The listing builds one solid part. Answer for the finished solid, in the listing's coordinates (mm). Give positions to 0.01 mm unless a question says otherwise; leave off trailing zeros. Order: outer loops, then holes, each group sorted by start corner. A loop starts at its lowest first (then second) coordinate and runs counter-clockwise, first axis right, second up. Notation, with made-up numbers: (54.5, 45) -> (88.5, 45) arc R23 cw to (88.5, 70) -> close; hole circle Ø6 at (82.5, 35.25). An arc over 180 degrees is marked (long way). Write item = value, one per line. Start each with the question number.
Autodesk Inventor part; units mm, degrees
ref_plane "YZ Plane" through (0, 0, 0) normal (1, 0, 0) x (0, 1, 0)
ref_plane "XZ Plane" through (0, 0, 0) normal (0, 1, 0) x (-1, 0, 0)
ref_plane "XY Plane" through (0, 0, 0) normal (0, 0, 1) x (1, 0, 0)
sketch "Sketch1" plane through (0, 0, 0) normal (0, 1, 0) x (-1, 0, 0)
  line L0 (-9.75, 149.5) -> (9.75, 149.5)
  line L1 (9.75, 149.5) -> (9.75, -149.5)
  line L2 (9.75, -149.5) -> (-9.75, -149.5)
  line L3 (-9.75, -149.5) -> (-9.75, 149.5)
  line L4 (-9.75, 149.5) -> (9.75, -149.5) construction
  line L5 (9.75, 149.5) -> (-9.75, -149.5) construction
  point P0 (0, 0)
  dimension "d0" = 19.5
  dimension "d1" = 299
extrude "Extrusion1" add sketch "Sketch1" along normal blind 5
chamfer "Chamfer1" distance 3 angle 45 1 edges at (-9.75, 5, 0)
sketch "Sketch2" plane through (-9.75, 0, 149.5) normal (0, 0, 1) x (1, 0, 0)
  line L0 (0, 2) -> (3, 5)
  line L1 (0, 0) -> (0, 2)
  line L2 (0, 0) -> (19.5, 0)
  line L3 (19.5, 0) -> (19.5, 5)
  line L4 (3, 5) -> (19.5, 5)
  line L5 (16.5, 4) -> (11.5, 4)
  line L6 (11.5, 4) -> (11.5, 1)
  line L7 (11.5, 1) -> (16.5, 1)
  line L8 (16.5, 1) -> (16.5, 4)
  line L9 (16.5, 4) -> (11.5, 1) construction
  line L10 (11.5, 4) -> (16.5, 1) construction
  point P0 (9.75, 0)
  point P1 (14, 2.5)
  point P2 (19.5, 2.5)
  dimension "d7" = 5
  dimension "d8" = 3
  dimension "d9" = 3
extrude "Extrusion2" cut sketch "Sketch2" against normal blind 7.1 contours L8 L7 L6 L5
sketch "Sketch3" plane through (9.75, 0, -149.5) normal (0, 0, -1) x (-1, 0, 0)
  line L0 (8, 1) -> (8, 4)
  line L1 (3, 1) -> (8, 1)
  line L2 (3, 4) -> (3, 1)
  line L3 (8, 4) -> (3, 4)
  line L4 (7.8, 1.2) -> (7.8, 3.8)
  line L5 (7.8, 3.8) -> (3.2, 3.8)
  line L6 (3.2, 3.8) -> (3.2, 1.2)
  line L7 (3.2, 1.2) -> (7.8, 1.2)
  point P0 (9.75, 0)
  dimension "d12" = 0.2
extrude "Extrusion3" add sketch "Sketch3" along normal blind 7 contours L7 L6 L5 L4
properties part number "SEPARADOR" material "Steel, Mild, Welded"
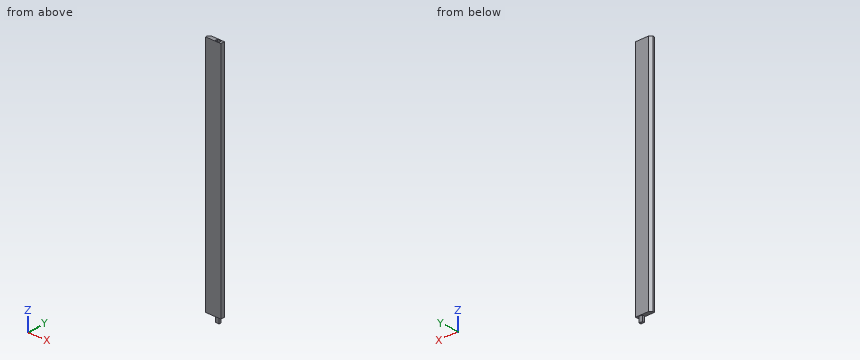
Item 1: A cutting plane is placed at B-B, the plane z = -105.5. Write down the section's boundary in (x, y).
Item 2: Consider L1, parallel to Z at x = -7.75, y = 3.3; L2, parallel to Z at x = 3, y = 1.3; L3, parallel to X at y = 3.1, z = 29.5. Determine where each line is inside the solid, lowest interval first. Write a range as from..to.
Item 3: Flat-ended cylindrical pins translate along their axes: pin 1 (2.5 mm diameter, centred on x = 5, z = -153.5, fed in from +Y); pin 2 (0.8 mm diameter, centred on y = 2, z = -152.5, fed in from -X); pin 3 (3 mm diameter, centred on y = 4, z = -19, fed in from -X). Find the tip coordinate at first contact, or state that the pin passes through.
Item 4: A cutting plane is placed at A-A, the plane y = 2.95. Write down the section's boundary in (x, z), plus the area to 3 significant figures.
Check values:
q1.outline = (-9.75, 0) -> (9.75, 0) -> (9.75, 5) -> (-6.75, 5) -> (-9.75, 2) -> close
q2.L1 = -149.5..149.5
q2.L2 = -156.5..142.4
q2.L3 = -8.65..9.75
q3.pin_1 = 3.8
q3.pin_2 = 1.95
q3.pin_3 = -9.25
q4.outline = (-8.8, -149.5) -> (1.95, -149.5) -> (1.95, -156.5) -> (6.55, -156.5) -> (6.55, -149.5) -> (9.75, -149.5) -> (9.75, 149.5) -> (6.75, 149.5) -> (6.75, 142.4) -> (1.75, 142.4) -> (1.75, 149.5) -> (-8.8, 149.5) -> close
q4.area = 5,540 mm^2
